```python
from build123d import *

# Parameters (mm, degrees)
SKETCH1_W           = 68.6
SKETCH1_H           = 53.3
BOSS_EXTRUDE1_DEPTH = 1.6
SKETCH2_W           = 15
SKETCH2_H           = 30.5
SKETCH2_W_2         = 10
SKETCH2_H_2         = 8.9
BOSS_EXTRUDE2_DEPTH = 10.9
SKETCH3_R           = 1.75
CUT_EXTRUDE1_DEPTH  = 2.6
SKETCH4_R           = 7.5
BOSS_EXTRUDE3_DEPTH = 14


with BuildPart() as part:
    # Sketch1 → Boss-Extrude1 (new body)
    with BuildSketch(Plane.XY):
        Rectangle(SKETCH1_W, SKETCH1_H)
    extrude(amount=BOSS_EXTRUDE1_DEPTH)

    # Sketch2 → Boss-Extrude2 (add)
    with BuildSketch(Plane.XY.offset(1.6)):
        with Locations((-33, 5.75)):
            Rectangle(SKETCH2_W, SKETCH2_H)
        with Locations((-16.3, -22.2)):
            Rectangle(SKETCH2_W_2, SKETCH2_H_2)
    extrude(amount=BOSS_EXTRUDE2_DEPTH)

    # Sketch3 → Cut-Extrude1 (cut, through all)
    with BuildSketch(Plane.XY.offset(1.6)):
        with Locations((-19, 24.05)):
            Circle(SKETCH3_R)
        with Locations((-20.3, -24.15)):
            Circle(SKETCH3_R)
        with Locations((31.8, -19.05)):
            Circle(SKETCH3_R)
        with Locations((31.8, 8.85)):
            Circle(SKETCH3_R)
    extrude(amount=-CUT_EXTRUDE1_DEPTH, mode=Mode.SUBTRACT)

    # Sketch4 → Boss-Extrude3 (add)
    with BuildSketch(Plane.XY.offset(1.6)):
        Circle(SKETCH4_R)
    extrude(amount=BOSS_EXTRUDE3_DEPTH)


solid = part.part
```
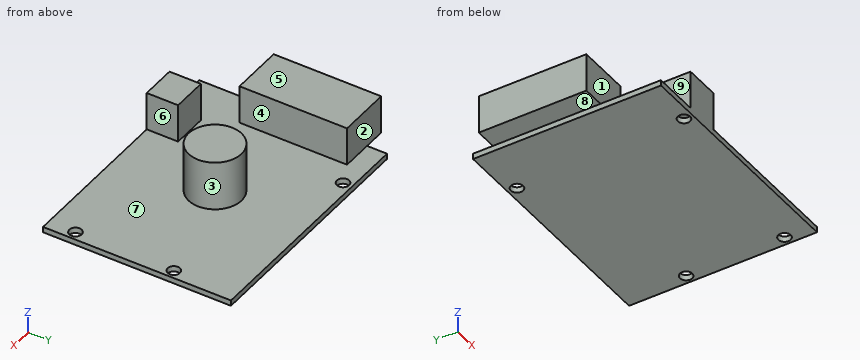
Check sheet for the modelled part. Datum: model origin and axes. Units: mm. Face numbers are marked on the shaded views. A direction names the side the tool comes from. Coordinates: 2 decimals unless noted, no trailing zeros. Order: outer loops, then holes, each group sorted by start corner. A loop starts at its lowest first (then second) coordinate and runs counter-clockwise, first axis right, second up. Notation, with made-up numbers: (88, -11.75) -> (137, -11.75) arc R17 ccw to (137, -6.75) -> close; hole circle Ø7 at (22, 60.5). An arc over 180 degrees is marked (long way). Write each question's results on one line, items separated by ' | '. Start each with the question number.
1) Set-up check for the marked faces 1, 2, 3, 4 and 5: record each of +Z, -Z, +X, -X, +Y, -Y from which the full face is reachable in a straight line by a thin tool's end or side.
2) Section check A-A (z = 9.25). Enter the section's corners in (x, y).
3) Draft check along X on the marked faces 6, 7, 8 and 9. Enter one of: pulls with the +X half, pulls with the -X half, needs draft (parallel to the pull), parting line crosses it, or undercut.
4) Section check B-B (y = 24.05). Enter the section's corners in (x, z), and give its area (3 significant figures).
5) Depth check by flat-ended pin: pin 1 (5 mm diameter, centred on y = 18.5, z = 7, fed in from +X); pin 2 (1.5 mm diameter, centred on x = 0.5, y = -19, fed in from +Z); pin 3 (8 mm diameter, centred on x = -16, z = 8.5, fed in from +Y). Enter the tip coordinate at first touch or a pass-through.
6) Section check C-C (x = 31.8). Enter the section's corners in (y, z), and give its area (3 significant figures).
7) Material ranges on line 1 along Y through (x, z) = (31.8, 0.3); line 2 along X through (y, z) = (-24.15, 0.4); line 3 along Z through (x, y) = (-28.5, 5), recorded low to high.
8) Section check D-D (x = 2). Enter the section's corners in (y, z).
Checked values:
1) face 1: +Z, +X, -X, -Y | face 2: +Z, +X, -X, +Y | face 3: +Z | face 4: +Z, +Y, -Y | face 5: +Z, -X, +Y, -Y
2) outline: (-40.5, -9.5) -> (-25.5, -9.5) -> (-25.5, 21) -> (-40.5, 21) -> close; (-21.3, -26.65) -> (-11.3, -26.65) -> (-11.3, -17.75) -> (-21.3, -17.75) -> close; circle Ø15 at (0, 0)
3) face 6: pulls with the +X half | face 7: undercut | face 8: needs draft | face 9: pulls with the -X half
4) outline: (-34.3, 0) -> (-20.75, 0) -> (-20.75, 1.6) -> (-34.3, 1.6) -> close; (-17.25, 0) -> (34.3, 0) -> (34.3, 1.6) -> (-17.25, 1.6) -> close | area: 104 mm²
5) pin 1: x = -25.5 | pin 2: z = 1.6 | pin 3: y = -17.75
6) outline: (-26.65, 0) -> (-20.8, 0) -> (-20.8, 1.6) -> (-26.65, 1.6) -> close; (-17.3, 0) -> (7.1, 0) -> (7.1, 1.6) -> (-17.3, 1.6) -> close; (10.6, 0) -> (26.65, 0) -> (26.65, 1.6) -> (10.6, 1.6) -> close | area: 74.1 mm²
7) line 1: -26.65 to -20.8, -17.3 to 7.1, 10.6 to 26.65 | line 2: -34.3 to -22.05, -18.55 to 34.3 | line 3: 0 to 12.5
8) outline: (-26.65, 0) -> (26.65, 0) -> (26.65, 1.6) -> (7.23, 1.6) -> (7.23, 15.6) -> (-7.23, 15.6) -> (-7.23, 1.6) -> (-26.65, 1.6) -> close
